The figure shows three views and two pictorial views of one solid part (mm, origin at its lowest corner). Answer the questions. Round coordinates to 2 decimals unless told otherwise and drop trailing zeros. Order: outer loops, then holes, each group sorted by start corner. A loop starts at its lowest first (then second) coordinate and runs counter-clockwise, first axis right, second up. Notation, with made-up numbers: (55, -40) -> (63, -40) arc R10 ccw to (63, -30) -> close; hole circle Ø5 at (54, 86.25). An arc over 180 degrees is marked (long way). Answer as a JSON object with one key per item and string values. Group by question number.
Item 1: Section B-B, the plane x = 114 is taken. Write down the section's boundary in (y, z), plus the area to 3 significant figures.
Item 2: Given P1, Ø12, axis at x = 91.5, z = 28, coming from the -Y side; P2, Ø1.5, axis at y = 2, z = 2, coming from the -X side; P3, Ø2.5, axis at x = 11, y = 3, coming from the +Z side; P4, Ø2.5, axis at y = 3.5, z = 3, coming from the +X side, each flat-ended and moving along its own axis, determine where each tip first touches the part or whether it passes through.
Item 3: Section C-C, the plane x = 43.5 is taken. Write down the section's boundary in (y, z).
Item 4: Section A-A, the plane y = 1.2 is taken. Write down the section's boundary in (x, z) (1 decimal).
Item 5: Consider probe 1 along X at (y, z) = (2.05, 44.5) (1 decimal); probe 2 along Z at (x, y) = (102, 3.2); probe 3 along Z at (x, y) = (87, 2.05). Determine where each line is inside the solid, lowest interval first. Write a range as from..to.
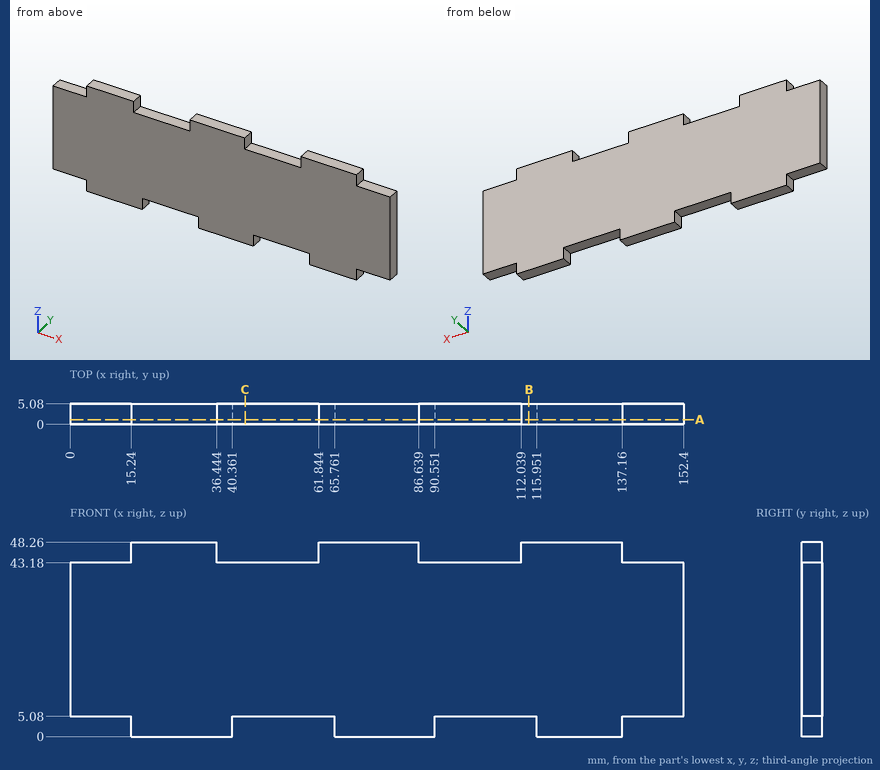
Values found:
{
 "1": {"outline": "(0, 5.08) -> (5.08, 5.08) -> (5.08, 48.26) -> (0, 48.26) -> close", "area": "219 mm2"},
 "2": {"P1": "y = 0", "P2": "x = 15.24", "P3": "z = 43.18", "P4": "x = 137.16"},
 "3": {"outline": "(0, 5.08) -> (5.08, 5.08) -> (5.08, 43.18) -> (0, 43.18) -> close"},
 "4": {"outline": "(0, 5.1) -> (15.2, 5.1) -> (15.2, 0) -> (40.4, 0) -> (40.4, 5.1) -> (65.8, 5.1) -> (65.8, 0) -> (90.6, 0) -> (90.6, 5.1) -> (116, 5.1) -> (116, 0) -> (137.2, 0) -> (137.2, 5.1) -> (152.4, 5.1) -> (152.4, 43.2) -> (137.2, 43.2) -> (137.2, 48.3) -> (112, 48.3) -> (112, 43.2) -> (86.6, 43.2) -> (86.6, 48.3) -> (61.8, 48.3) -> (61.8, 43.2) -> (36.4, 43.2) -> (36.4, 48.3) -> (15.2, 48.3) -> (15.2, 43.2) -> (0, 43.2) -> close"},
 "5": {"probe 1": "15.2..36.4, 61.8..86.6, 112..137.2", "probe 2": "5.08..43.18", "probe 3": "0..43.18"}
}
